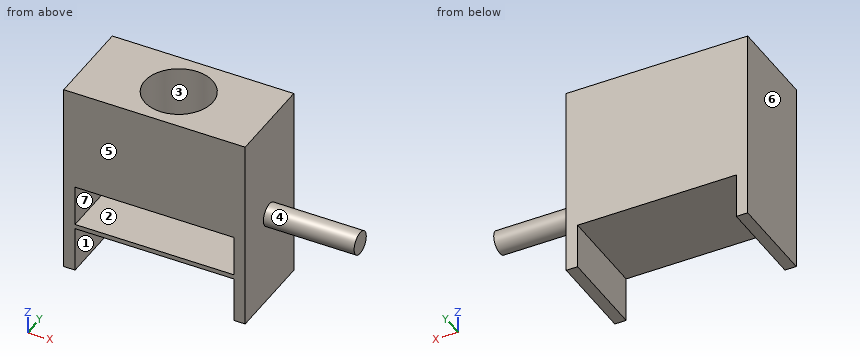
from build123d import *

# Parameters (mm, degrees)
F0_W     = 44.45
F0_H     = 1.27
F1_DEPTH = 25.4
F2_R     = 9.525
F3_DEPTH = 38.1
F4_W     = 1.27
F4_H     = 11.43
F5_DEPTH = 44.45
F6_R     = 3.175
F7_DEPTH = 25.4


with BuildPart() as f1:
    # F0 (on Front) → F1 (new body)
    with BuildSketch(Plane.XZ):
        Polygon((-22.225, -11.43), (-22.225, 0), (-25.4, 0), (-25.4, -25.4), (-22.225, -25.4), (-22.225, -12.7), align=None)
        Polygon((25.4, 0), (22.225, 0), (22.225, -11.43), (22.225, -12.7), (22.225, -25.4), (25.4, -25.4), align=None)
        Polygon((-22.225, 0), (0, 0), (22.225, 0), (25.4, 0), (25.4, 28.7261897342), (-25.4, 28.7261897342), (-25.4, 0), align=None)
        with Locations((0, -12.065)):
            Rectangle(F0_W, F0_H)
    extrude(amount=F1_DEPTH)

    # F2 (on face) → F3 (cut)
    with BuildSketch(Plane.XY.offset(28.7261897342)):
        with Locations((0, -12.7)):
            Circle(F2_R)
    extrude(amount=-F3_DEPTH, mode=Mode.SUBTRACT)

    # F4 (on face) → F5 (join)
    with BuildSketch(Plane.YZ.offset(-22.225)):
        with Locations((-0.635, -5.715)):
            Rectangle(F4_W, F4_H)
    extrude(amount=F5_DEPTH)

    # F6 (on face) → F7 (join)
    with BuildSketch(Plane.YZ.offset(25.4)):
        with Locations((-12.7, 0)):
            Circle(F6_R)
    extrude(amount=F7_DEPTH)


solid = f1.part
Here's how the part is built. I have some questions about the finished solid (model axes, mm). Face numbers are marked on the shaded views. A direction names the side the tool comes from. Give positions to 0.01 mm unless a question says otherwise; leave off trailing zeros. Order: outer loops, then holes, each group sorted by start corner. A loop starts at its lowest first (then second) coordinate and runs counter-clockwise, first axis right, second up. Notation, with made-up numbers: (0.5, -7) -> (11.5, -7) arc R16 cw to (11.5, 20) -> close; hole circle Ø10 at (58.5, 77.5). An arc over 180 degrees is marked (long way). Use a Markdown table: item, result. Add a question column.
Item 1: I need wall thicknesses on line 1 (X direction, y = -10.25, z = -21) (3 decimals); line 2 (Z direction, x = -8.5, y = -18.25); line 3 (Y direction, x = 0, z = 16) (3 decimals). Which ranges of each line are inside material? Lowest first, please.
Item 2: If we mould it in two halves opening along X, with no side actions, what happens to the marked faces 5, 6 and 7? For each: pulls with the +X half, pulls with the -X half, needs draft (parallel to the pull), parting line crosses it, or undercut.
Item 3: Imagine slicing it at A-A on z = -20. Please give me the cut outline in (x, y) (3 decimals).
Item 4: Imagine slicing it at D-D on z = 9. Please give me the cut outline in (x, y) (3 decimals).
Item 5: Imagine slicing it at C-C on y = -23. Please give me the cut outline in (x, z) (3 decimals), plus the area to 3 significant figures.
Item 6: Imagine slicing it at B-B on x = 0. Please give me the cut outline in (y, z) (3 decimals).
Item 7: Will these pins go through, and if not, where does the flat tip stop? pin 1 (3.5 mm diameter, centred on x = -7.5, z = -5, fed in from -Y); pin 2 (1 mm diameter, centred on x = 21, z = -15.5, fed in from +Y); pin 3 (6 mm diameter, centred on x = -3, y = -14, fed in from -Z); pin 4 (12 mm diameter, centred on y = -4.5, z = 20, fed in from +X).
Item 8: For the marked faces 1, 2, 3 and 4, which set-ups out of +Z, -Z, +X, -X, +Y, -Y let a thin tool reach every point of the face, with its end or its side?
Data:
| question | item | result |
|---|---|---|
| 1 | line 1 | x = -25.4 to -22.225, 22.225 to 25.4 |
| 1 | line 2 | z = -12.7 to -11.43, 0 to 28.73 |
| 1 | line 3 | y = -25.4 to -22.225, -3.175 to 0 |
| 2 | face 5 | needs draft |
| 2 | face 6 | pulls with the -X half |
| 2 | face 7 | undercut |
| 3 | outline | (-25.4, -25.4) -> (-22.225, -25.4) -> (-22.225, 0) -> (-25.4, 0) -> close; (22.225, -25.4) -> (25.4, -25.4) -> (25.4, 0) -> (22.225, 0) -> close |
| 4 | outline | (-25.4, -25.4) -> (25.4, -25.4) -> (25.4, 0) -> (-25.4, 0) -> close; hole circle Ø19.05 at (0, -12.7) |
| 5 | outline | (-25.4, -25.4) -> (-22.225, -25.4) -> (-22.225, -12.7) -> (22.225, -12.7) -> (22.225, -25.4) -> (25.4, -25.4) -> (25.4, 28.726) -> (-25.4, 28.726) -> close; hole (-22.225, -11.43) -> (22.225, -11.43) -> (22.225, 0) -> (-22.225, 0) -> close |
| 5 | area | 1,680 mm² |
| 6 | outline | (-25.4, -12.7) -> (0, -12.7) -> (0, 28.726) -> (-3.175, 28.726) -> (-3.175, 0) -> (-1.27, 0) -> (-1.27, -11.43) -> (-25.4, -11.43) -> close; (-25.4, 0) -> (-22.225, 0) -> (-22.225, 28.726) -> (-25.4, 28.726) -> close |
| 7 | pin 1 | stops at y = -1.27 |
| 7 | pin 2 | passes through |
| 7 | pin 3 | stops at z = -12.7 |
| 7 | pin 4 | stops at x = 25.4 |
| 8 | face 1 | -Z, +Y, -Y |
| 8 | face 2 | -Y |
| 8 | face 3 | +Z |
| 8 | face 4 | +X |
